Check sheet for the modelled part. Datum: model origin and axes. Units: mm. Face numbers are marked on the shaded views. A direction names the side the tool comes from. Give positions to 0.01 mm unless a question says otherwise; leave off trailing zeros. Order: outer loops, then holes, each group sorted by start corner. A loop starts at its lowest first (then second) coordinate and runs counter-clockwise, first axis right, second up.
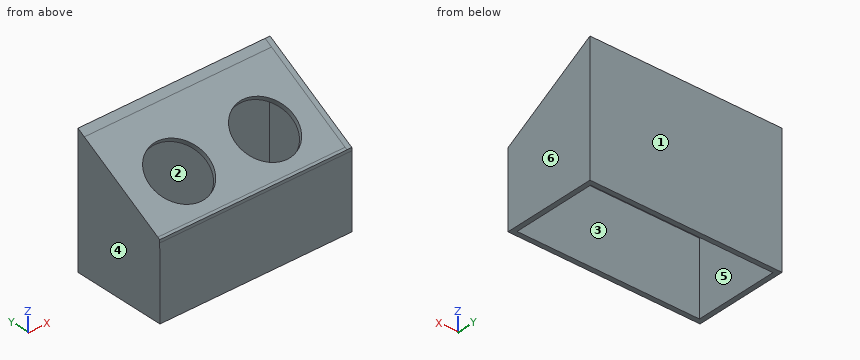
Autodesk Fusion 360 part; units mm, degrees
sketch "Sketch1" plane through (0, 0, 0) normal (1, 0, 0) x (0, 0, -1)
  line L0 (0, 0) -> (-20, 34.641)
  line L1 (0, 0) -> (40, 0) construction
  line L2 (-20, 34.641) -> (30, 34.641)
  line L3 (30, 34.641) -> (30, 0)
  line L4 (30, 0) -> (0, 0)
  dimension "d1" = 120
  dimension "d2" = 40
  dimension "d3" = 50
extrude "Extrude1" add sketch "Sketch1" against normal blind 2
sketch "Sketch2" plane through (0, 0, 0) normal (1, 0, 0) x (0, 0, -1)
  line L0 (0, 0) -> (2, 0) construction
  line L1 (30, 0) -> (30, 34.641)
  line L2 (30, 34.641) -> (-20, 34.641)
  line L3 (-20, 34.641) -> (0, 0)
  line L4 (0, 0) -> (30, 0)
  line L5 (-20, 34.641) -> (-18, 34.641) construction
  line L6 (30, 0) -> (30, -2)
  line L7 (30, 34.641) -> (30, 36.641)
  line L8 (30, 36.641) -> (-23.4641, 36.641)
  line L9 (-1.7321, -1) -> (-21.7321, 33.641)
  line L10 (30, -2) -> (0, -1.8905)
  line L11 (-21.7321, 33.641) -> (-23.4641, 36.641)
  line L12 (0, -1.8905) -> (-1.2179, -1.8905)
  line L13 (-1.7321, -1) -> (-1.2179, -1.8905)
  line L14 (30, 0) -> (0, 0)
  line L15 (-20, 34.641) -> (30, 34.641)
  dimension "d7" = 2
  dimension "d10" = 2
  dimension "d12" = 2
  dimension "d13" = 2
extrude "Extrude2" add sketch "Sketch2" against normal blind 2 contours L2 L3 L4 L6 L7 L8 L9 L10 L11 L12 L13 L14 L15
extrude "Extrude3" add sketch "Sketch2" along normal blind 75 contours L2 L3 L4 L6 L7 L8 L9 L10 L11 L12 L13 L14 L15
sketch "Sketch3" plane through (75, 0, 0) normal (1, 0, 0) x (0, 0, -1)
  line L0 (30, 34.641) -> (30, 36.641)
  line L1 (30, 36.641) -> (-23.4641, 36.641)
  line L2 (-23.4641, 36.641) -> (-1.2179, -1.8905)
  line L3 (-1.2179, -1.8905) -> (0, -1.8905)
  line L4 (0, -1.8905) -> (30, -2)
  line L5 (30, -2) -> (30, 0)
  line L6 (-23.4641, 36.641) -> (30, 36.641)
  line L7 (30, -2) -> (-1.2179, -1.8905)
  line L8 (30, 0) -> (0, 0)
  line L9 (0, 0) -> (-20, 34.641)
  line L10 (-20, 34.641) -> (30, 34.641)
  line L11 (30, 34.641) -> (30, 36.641)
  line L12 (30, 36.641) -> (-23.4641, 36.641)
  line L13 (-23.4641, 36.641) -> (-1.2179, -1.8905)
  line L14 (-1.2179, -1.8905) -> (0, -1.8905)
  line L15 (0, -1.8905) -> (30, -2)
  line L16 (30, -2) -> (30, 0)
  line L17 (30, -2) -> (30, 36.641)
  line L18 (30, 36.641) -> (-23.4641, 36.641)
  line L19 (-23.4641, 36.641) -> (-1.2179, -1.8905)
  line L20 (-1.2179, -1.8905) -> (30, -2)
extrude "Extrude4" add sketch "Sketch3" along normal blind 2 contours L0 L1 L2 L3 L4 L5 L6 L8 L9 L10 L11 L12 L13 L14 L15 L16 L17 L18 L19 | L8 L9 L10 L17
hole "Hole1" at (19.1728, 13.2188, 9.9413) direction (0, 0.5, -0.866) diameter 24 depth 20 tip angle 118
hole "Hole2" at (54.6679, 13.3913, 10.0409) direction (0, 0.5, -0.866) diameter 24 depth 20 tip angle 118
(1) Sectioned sample at A-A (x = 39). Enter the section's corners in (y, z), plus the area to 3 significant figures.
(2) Sectioned sample at D-D (y = 32.5). Enter the section's corners in (x, z), plus the area to 3 significant figures.
(3) Release check for a two-part mould opening along Y. For the marked faces 1, 2, 3 and 4 record: released by +Y, released by -Y, zero draft, split by the parting line, or undercut.
(4) Sectioned sample at B-B (x = 23.5). Enter the section's corners in (y, z) (1 decimal).
(5) Go/stop test with flat-tipped pins: P1, Ø12, axis at x = 32, y = 28.5, coming from the +Z side; P2, Ø10, axis at x = 53.5, z = 4.5, coming from the -Y side; P3, Ø4, axis at x = 58.5, y = 25.5, coming from the -Z side. Record where each tip stops, or that it passes through.
(6) Sectioned sample at C-C (z = -18.5). Enter the section's corners in (x, y), plus the area to 3 significant figures.
(7) Thickness scan on L1, parallel to X at y = 28.5, z = -5.5; L2, parallel to Y at x = 72, z = -3; L3, parallel to X at y = 9, z = 7. Record the ranges inside material, lowest first.
(8) Tool access check on the marked faces 5 and 6. Record the directions out of +Z, -Z, +X, -X, +Y, -Y that give a thin tool (end or side, any length) a straight path to the whole face; none if there is none.
Values follow:
1. outline: (-2, -30) - (0, -30) - (0, 0) - (34.64, 20) - (34.64, -30) - (36.64, -30) - (36.64, 23.46) - (33.64, 21.73) - (-1, 1.73) - (-1.89, 1.22) - (-1.89, 0) - close
1. area: 247 mm2
2. outline: (-2, -30) - (0, -30) - (0, 18.76) - (75, 18.76) - (75, -30) - (77, -30) - (77, 21.07) - (-2, 21.07) - close
2. area: 378 mm2
3. face 1: released by +Y
3. face 2: undercut
3. face 3: undercut
3. face 4: zero draft
4. outline: (-2, -30) - (0, -30) - (0, 0) - (4.5, 2.6) - (3.5, 4.3) - (-1, 1.7) - (-1.9, 1.2) - (-1.9, 0) - close; (22.9, 15.5) - (23.9, 13.8) - (34.6, 20) - (34.6, -30) - (36.6, -30) - (36.6, 23.5) - (33.6, 21.7) - close
5. P1: stops at z = 22.23
5. P2: stops at y = -1.89
5. P3: stops at z = 13.77
6. outline: (-2, -1.96) - (77, -1.96) - (77, 36.64) - (-2, 36.64) - close; hole (0, 0) - (75, 0) - (75, 34.64) - (0, 34.64) - close
6. area: 451 mm2
7. L1: x = -2 to 0, 75 to 77
7. L2: y = -1.9 to 0, 34.64 to 36.64
7. L3: x = -2 to 8.32, 30.02 to 43.91, 65.42 to 77
8. face 5: -Z
8. face 6: +Z, -Z, +X, +Y, -Y
